```python
from build123d import *

# Parameters (mm, degrees)
F0_R     = 0.75
F1_DEPTH = 1


# Not quite as in the source:
# - a feature names something its author has since deleted; it is built from what else it names


with BuildPart() as f1:
    # F0 (on Right) → F1 (new body)
    with BuildSketch(Plane.YZ):
        Polygon((8.384144865, 0), (0, 0), (0, -11.5), (11.5, -11.5), (11.5, 0), (10.384144865, 0), (10.384144865, 10), (8.384144865, 10), align=None)
        with Locations((1.75, -9.75)):
            Circle(F0_R, mode=Mode.SUBTRACT)
        with Locations((1.75, -7.75)):
            Circle(F0_R, mode=Mode.SUBTRACT)
        with Locations((3.75, -9.75)):
            Circle(F0_R, mode=Mode.SUBTRACT)
        with Locations((3.75, -7.75)):
            Circle(F0_R, mode=Mode.SUBTRACT)
        with Locations((1.75, -5.75)):
            Circle(F0_R, mode=Mode.SUBTRACT)
        with Locations((1.75, -3.75)):
            Circle(F0_R, mode=Mode.SUBTRACT)
        with Locations((1.75, -1.75)):
            Circle(F0_R, mode=Mode.SUBTRACT)
        with Locations((3.75, -5.75)):
            Circle(F0_R, mode=Mode.SUBTRACT)
        with Locations((3.75, -3.75)):
            Circle(F0_R, mode=Mode.SUBTRACT)
        with Locations((3.75, -1.75)):
            Circle(F0_R, mode=Mode.SUBTRACT)
        with Locations((5.75, -9.75)):
            Circle(F0_R, mode=Mode.SUBTRACT)
        with Locations((7.75, -9.75)):
            Circle(F0_R, mode=Mode.SUBTRACT)
        with Locations((5.75, -7.75)):
            Circle(F0_R, mode=Mode.SUBTRACT)
        with Locations((7.75, -7.75)):
            Circle(F0_R, mode=Mode.SUBTRACT)
        with Locations((9.75, -9.75)):
            Circle(F0_R, mode=Mode.SUBTRACT)
        with Locations((9.75, -7.75)):
            Circle(F0_R, mode=Mode.SUBTRACT)
        with Locations((5.75, -5.75)):
            Circle(F0_R, mode=Mode.SUBTRACT)
        with Locations((5.75, -3.75)):
            Circle(F0_R, mode=Mode.SUBTRACT)
        with Locations((7.75, -5.75)):
            Circle(F0_R, mode=Mode.SUBTRACT)
        with Locations((7.75, -3.75)):
            Circle(F0_R, mode=Mode.SUBTRACT)
        with Locations((5.75, -1.75)):
            Circle(F0_R, mode=Mode.SUBTRACT)
        with Locations((7.75, -1.75)):
            Circle(F0_R, mode=Mode.SUBTRACT)
        with Locations((9.75, -5.75)):
            Circle(F0_R, mode=Mode.SUBTRACT)
        with Locations((9.75, -3.75)):
            Circle(F0_R, mode=Mode.SUBTRACT)
        with Locations((9.75, -1.75)):
            Circle(F0_R, mode=Mode.SUBTRACT)
    extrude(amount=F1_DEPTH)


solid = f1.part
```
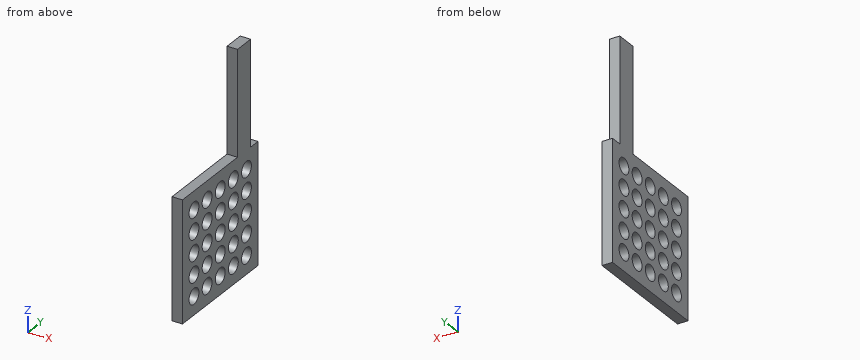
Geometry check sheet. Reference: the model listing, model coordinates, mm. Give positions to 0.01 mm unless a question says otherwise; leave off trailing zeros. Order: outer loops, then holes, each group sorted by start corner. A loop starts at its lowest first (then second) coordinate and runs counter-clockwise, first axis right, second up. Notation, with made-up numbers: (-35, 65) - (-30, 65) arc R18 cw to (-30, 84) - close; hole circle Ø7 at (29, 21). An arc over 180 degrees is marked (long way). Answer in a Markdown table with one row per item. Add a question column.
Q1. Cross-section at C-C, the plane x = 0.3. Count the separate pieces of the cut face and the enclosed holes in it, then the cut area to 3 significant figures.
Q2. Cross-section at B-B, the plane z = -7.25. Enter the section's corners in (x, y), then the cut area to 3 significant figures.
Q3. Cross-section at A-A, the plane y = 5.75. Enter the section's corners in (x, z).
Q4. Gauge pin test, flat end, axial feed: pin 1 (0.5 mm diameter, centred on x = 0.5, z = 4.5, fed in from +Y). Record the tip position at first contact, or that the pin passes through.
Q5. Cross-section at D-D, the plane z = 2.25. Enter the section's corners in (x, y).
Q6. Material ranges on probe 1 along Z at (x, y) = (0.35, 3.75); probe 2 along Z at (x, y) = (0.5, 9.75); probe 3 along Y at (x, z) = (0.4, -6.25), recorded low to high. Write a range as from..to.
Check values:
| question | item | result |
|---|---|---|
| 1 | separate pieces | 1 |
| 1 | enclosed holes | 25 |
| 1 | area | 108 mm^2 |
| 2 | outline | (0, 0) - (1, 0) - (1, 1.19) - (0, 1.19) - close; (0, 2.31) - (1, 2.31) - (1, 3.19) - (0, 3.19) - close; (0, 4.31) - (1, 4.31) - (1, 5.19) - (0, 5.19) - close; (0, 6.31) - (1, 6.31) - (1, 7.19) - (0, 7.19) - close; (0, 8.31) - (1, 8.31) - (1, 9.19) - (0, 9.19) - close; (0, 10.31) - (1, 10.31) - (1, 11.5) - (0, 11.5) - close |
| 2 | area | 5.91 mm^2 |
| 3 | outline | (0, -11.5) - (1, -11.5) - (1, -10.5) - (0, -10.5) - close; (0, -9) - (1, -9) - (1, -8.5) - (0, -8.5) - close; (0, -7) - (1, -7) - (1, -6.5) - (0, -6.5) - close; (0, -5) - (1, -5) - (1, -4.5) - (0, -4.5) - close; (0, -3) - (1, -3) - (1, -2.5) - (0, -2.5) - close; (0, -1) - (1, -1) - (1, 0) - (0, 0) - close |
| 4 | pin 1 | stops at y = 10.38 |
| 5 | outline | (0, 8.38) - (1, 8.38) - (1, 10.38) - (0, 10.38) - close |
| 6 | probe 1 | z = -11.5..-10.5, -9..-8.5, -7..-6.5, -5..-4.5, -3..-2.5, -1..0 |
| 6 | probe 2 | z = -11.5..-10.5, -9..-8.5, -7..-6.5, -5..-4.5, -3..-2.5, -1..10 |
| 6 | probe 3 | y = 0..1.19, 2.31..3.19, 4.31..5.19, 6.31..7.19, 8.31..9.19, 10.31..11.5 |
